```python
from build123d import *

# Parameters (mm, degrees)
SKETCH1_W           = 137
SKETCH1_H           = 44
BOSS_EXTRUDE1_DEPTH = 18
FILLET1_R           = 6
FILLET2_R           = 2
SKETCH2_R           = 2.5
BOSS_EXTRUDE2_DEPTH = 2


with BuildPart() as part:
    # Sketch1 → Boss-Extrude1 (new body)
    with BuildSketch(Plane(origin=(0, 0, 0), x_dir=(0, 1, 0), z_dir=(0, 0, 1))):
        Rectangle(SKETCH1_W, SKETCH1_H)
    extrude(amount=BOSS_EXTRUDE1_DEPTH)

    # Fillet1
    fillet1_edges = [part.edges().sort_by_distance(p)[0] for p in [
        (0, -68.5, 18),
        (0, -68.5, 0),
    ]]
    fillet(fillet1_edges, radius=FILLET1_R)

    # Fillet2
    fillet2_edges = [part.edges().sort_by_distance(p)[0] for p in [
        (22, -68.5, 9),
        (-22, -68.5, 9),
        (22, 3, 0),
        (22, 3, 18),
        (22, -66.742640687, 16.242640687),
        (22, -66.742640687, 1.757359313),
        (-22, -66.742640687, 16.242640687),
        (-22, -66.742640687, 1.757359313),
        (0, 68.5, 18),
        (-22, 3, 0),
        (0, 68.5, 0),
        (22, 68.5, 9),
        (-22, 68.5, 9),
        (-22, 3, 18),
    ]]
    fillet(fillet2_edges, radius=FILLET2_R)

    # Sketch2 → Boss-Extrude2 (add)
    with BuildSketch(Plane(origin=(-22, 0, 0), x_dir=(0, -1, 0), z_dir=(-1, 0, 0))):
        with Locations(Location((62.5, 12.5, 0), (0, 0, 270))):
            Circle(SKETCH2_R)
        with Locations(Location((62.5, 5.5, 0), (0, 0, 270))):
            Circle(SKETCH2_R)
    extrude(amount=BOSS_EXTRUDE2_DEPTH)


solid = part.part
```
The listing builds one solid part. Answer for the finished solid, in the listing's coordinates (mm). A direction names the side the tool comes from. Round coordinates to 2 decimals unless told otherwise and drop trailing zeros. Loops run counter-clockwise (first coordinate to the right, second up) from the corner with the lowest first, then second, coordinate; pieces in that order, holes last. Notation, with made-up numbers: (18.25, -34.5) - (42.25, -34.5) arc R22 ccw to (42.25, -17.5) - close; hole circle Ø9 at (-10.5, 44). An arc over 180 degrees is marked (long way). Use one line per item in the form item = value. Start each with the question number.
1. Consider line 1 (X direction, y = 57, z = 11.25); line 2 (Y direction, x = 20.5, z = 17); line 3 (X direction, y = -56, z = 16.5). Determine where each line is inside the solid, lowest interval first. Write a range as [from, to].
2. For a pull along Z with two mould halves and no side action, classify faces 1 (the face through (-22.986, -63.251, 3.115)), 2 (the face through (0, 1, 18)), 3 (the face through (-24, -63, 6)) as pulls with the +Z half, pulls with the -Z half, needs draft (parallel to the pull), parting line crosses it, or undercut.
3. The part is cut by section A-A on y = -3. Determine the outline of the cut face in (x, z), then the cut area to 3 significant figures.
4. A tool of negligible diameter and unlimited length cuts with its end or side. For faces 4 (the face through (-0.28, -66.789, 16.196)), 5 (the face through (-23, -62.6, 15)), from which of +Z, -Z, +X, -X, +Y, -Y can it reach the whole face along a straight path? Write none if from no direction.
Geometry check:
q1.line_1 = [-22, 22]
q1.line_2 = [-65.7, 68.16]
q1.line_3 = [-21.94, 21.94]
q2.face_1 = undercut
q2.face_2 = pulls with the +Z half
q2.face_3 = needs draft
q3.outline = (-22, 2) arc R2 ccw to (-20, 0) - (20, 0) arc R2 ccw to (22, 2) - (22, 16) arc R2 ccw to (20, 18) - (-20, 18) arc R2 ccw to (-22, 16) - close
q3.area = 789 mm^2
q4.face_4 = +Z, +X, -X, -Y
q4.face_5 = -X
